Autodesk Inventor part; units mm, degrees
ref_plane "YZ Plane" through (0, 0, 0) normal (1, 0, 0) x (0, 1, 0)
ref_plane "XZ Plane" through (0, 0, 0) normal (0, 1, 0) x (-1, 0, 0)
ref_plane "XY Plane" through (0, 0, 0) normal (0, 0, 1) x (1, 0, 0)
sketch "Sketch1" plane through (0, 0, 0) normal (0, 0, 1) x (1, 0, 0)
  line L0 (-72, 72) -> (72, 72)
  line L1 (72, 72) -> (72, -72)
  line L2 (72, -72) -> (-72, -72)
  line L3 (-72, -72) -> (-72, 72)
  line L4 (20, 55) -> (50, 55)
  line L5 (50, 55) -> (50, 25)
  line L6 (50, 25) -> (20, 25)
  line L7 (20, 25) -> (20, 55)
  point P0 (0, 0)
  dimension "d0" = 144
  dimension "d1" = 144
  dimension "d2" = 72
  dimension "d3" = 72
  dimension "d4" = 20
  dimension "d5" = 25
  dimension "d6" = 30
  dimension "d7" = 30
extrude "Extrusion1" add sketch "Sketch1" along normal blind 5
fillet "Fillet1" radius 5 4 edges at (-72, -72, 2.5) (72, -72, 2.5) (72, 72, 2.5) (-72, 72, 2.5)
sketch "Sketch3" plane through (0, 0, 5) normal (0, 0, 1) x (1, 0, 0)
  line L0 (-59.5, 59.5) -> (59.5, 59.5)
  line L1 (59.5, 59.5) -> (59.5, -59.5)
  line L2 (59.5, -59.5) -> (-59.5, -59.5)
  line L3 (-59.5, -59.5) -> (-59.5, 59.5)
  circle A0 centre (-59.5, 59.5) radius 3
  point P0 (0, 0)
  dimension "d23" = 119
  dimension "d24" = 119
  dimension "d25" = 59.5
  dimension "d26" = 59.5
  dimension "d27" = 6
hole "Hole2" at (-59.5, 59.5, 5) at (59.5, 59.5, 5) at (59.5, -59.5, 5) at (-59.5, -59.5, 5) direction (0, 0, -1) diameter 6 end through all
equation "\"d28\" = d27"
properties part number "WaagePlexiTurm" material "PET Plastic"
Can you work these out from the model? Positions are in its coordinate system, mm. A direction names the side the tool comes from. Round coordinates to 2 decimals unless told otherwise and drop trailing zeros. Loops run counter-clockwise (first coordinate to the right, second up) from the corner with the lowest first, then second, coordinate; pieces in that order, holes last. Notation, with made-up numbers: (43, -24.5) -> (67, -24.5) arc R22 ccw to (67, 14.5) -> close; hole circle Ø6 at (9.5, 41). An arc over 180 degrees is marked (long way). One line per item, written item: value. Start each with the question number.
1. If we mould it in two halves opening along X, with no side actions, what happens to faces 1 (the flat face through (-1, 72, 2)), 2 (the cylindrical face through (70, -71, 3)), 3 (the cylindrical face through (-71, -70, 3)), 4 (the cylindrical face through (-61.53, 61.71, 2.46))? For each: pulls with the +X half, pulls with the -X half, needs draft (parallel to the pull), parting line crosses it, or undercut.
2. If I drill on probe 1 along X at (y, z) = (-59.5, 2.2); probe 2 along Y at (x, z) = (21, 0.4), over which ranges is the centre line in solid material (lowest first)?
3. For pin 1 (5.5 mm diameter, centred on x = 59.5, y = -59.5, fed in from +Z) (3 decimals), with a flat end and sliding along its axis, tell me the tip position at first contact or that it passes through.
4. If we section it at A-A, the plane y = 59.5: Write out the boundary of the cut face in (x, z).
5. If we section it at C-C, the plane z = 0.95: Write out the boundary of the cut face in (x, y).
6. For faces 5 (the flat face through (1, -72, 2)), 6 (the flat face through (20, 40, 2)), which set-ups out of +Z, -Z, +X, -X, +Y, -Y let a thin tool reach every point of the face, with its end or its side?
Calculated:
1. face 1: needs draft
1. face 2: pulls with the +X half
1. face 3: pulls with the -X half
1. face 4: undercut
2. probe 1: x = -72 to -62.5, -56.5 to 56.5, 62.5 to 72
2. probe 2: y = -72 to 25, 55 to 72
3. pin 1: passes through
4. outline: (-72, 0) -> (-62.5, 0) -> (-62.5, 5) -> (-72, 5) -> close; (-56.5, 0) -> (56.5, 0) -> (56.5, 5) -> (-56.5, 5) -> close; (62.5, 0) -> (72, 0) -> (72, 5) -> (62.5, 5) -> close
5. outline: (-72, -67) arc R5 ccw to (-67, -72) -> (67, -72) arc R5 ccw to (72, -67) -> (72, 67) arc R5 ccw to (67, 72) -> (-67, 72) arc R5 ccw to (-72, 67) -> close; hole circle Ø6 at (-59.5, -59.5); hole circle Ø6 at (-59.5, 59.5); hole (20, 25) -> (50, 25) -> (50, 55) -> (20, 55) -> close; hole circle Ø6 at (59.5, -59.5); hole circle Ø6 at (59.5, 59.5)
6. face 5: +Z, -Z, +X, -X, -Y
6. face 6: +Z, -Z
